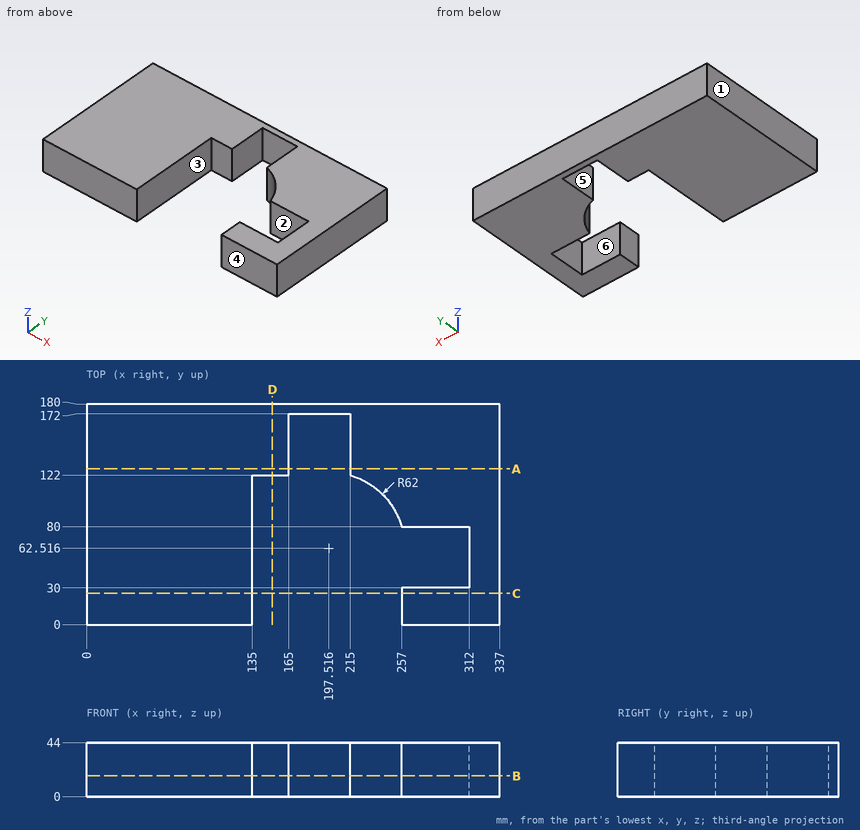
Input: dimensioned drawing with shaded views. Units: mm. Origin: part minimum x, y, z. A direction names the side the tool comes from. Coordinates: 2 decimals unless noted, no trailing zeros. Loops run counter-clockwise (first coordinate to the right, second up) from the corner with the lowest first, then second, coordinate; pieces in that order, holes last. Notation, with made-up numbers: (-23.5, 71.5) -> (-18.5, 71.5) arc R35 ccw to (-18.5, 104.5) -> close; hole circle Ø9 at (0, 63.5). An arc over 180 degrees is marked (long way). Use a Markdown table: item, result. Add a question column.
(1) Section query B-B, the plane z = 17. Return loops of the section in (x, y).
(2) Access query for the marked faces 1, 2 and 3. Directions: +Z, -Z, +X, -X, +Y, -Y. A direction counts if a zero-diameter tool reaches every point of the face in a straight line with its end or side. Return the directions, or none.
(3) Section query A-A, the plane y = 127. Return loops of the section in (x, z), plus the area to 3 significant figures.
(4) Line query: line 1 along X through (y, z) = (132, 23); line 2 along X through (y, z) = (58.5, 35); line 3 along Y through (x, z) = (144, 15). Output: solid intervals per line, ascending.
(5) Mould query, pull axis Y, two halves, no side actions, for the marked faces 4, 5 and 6. Classes: pulls with the +Y half, pulls with the -Y half, needs draft (parallel to the pull), parting line crosses it, or undercut.
(6) Section query C-C, the plane y = 25.5. Return loops of the section in (x, z).
(7) Section query D-D, the plane x = 151.5. Return loops of the section in (y, z), plus the area to 3 significant figures.
(8) Pin query (flat end, axial travel): pin 1 Ø15 at (x, z) = (151, 32.5) entering from -Y. Return the tip coordinate at first contact, or that it passes through.
Answer:
| question | item | result |
|---|---|---|
| 1 | outline | (0, 0) -> (135, 0) -> (135, 122) -> (165, 122) -> (165, 172) -> (215, 172) -> (215, 122) arc R62 cw to (257, 80) -> (312, 80) -> (312, 30) -> (257, 30) -> (257, 0) -> (337, 0) -> (337, 180) -> (0, 180) -> close |
| 2 | face 1 | +Z, -Z, -X, +Y, -Y |
| 2 | face 2 | +Z, -Z |
| 2 | face 3 | +Z, -Z, -Y |
| 3 | outline | (0, 0) -> (165, 0) -> (165, 44) -> (0, 44) -> close; (215, 0) -> (337, 0) -> (337, 44) -> (215, 44) -> close |
| 3 | area | 12,600 mm^2 |
| 4 | line 1 | x = 0 to 165, 215 to 337 |
| 4 | line 2 | x = 0 to 135, 312 to 337 |
| 4 | line 3 | y = 122 to 180 |
| 5 | face 4 | pulls with the -Y half |
| 5 | face 5 | needs draft |
| 5 | face 6 | undercut |
| 6 | outline | (0, 0) -> (135, 0) -> (135, 44) -> (0, 44) -> close; (257, 0) -> (337, 0) -> (337, 44) -> (257, 44) -> close |
| 7 | outline | (122, 0) -> (180, 0) -> (180, 44) -> (122, 44) -> close |
| 7 | area | 2,550 mm^2 |
| 8 | pin 1 | stops at y = 122 |
